Solid Edge part; units mm, degrees
sketch "Sketch1" plane through (0, 0, 0) normal (0, 0, 1) x (1, 0, 0)
  line L0 (-2.5, -5.2) -> (-8.5417, -5.2)
  line L1 (-5, -8.6603) -> (-8.75, -15.1554)
  line L2 (-5, 8.6603) -> (-8.75, 15.1554)
  arc A0 (-8.5417, 5.2) -> (-5, 8.6603) centre (0, 0) cw
  line L3 (-2.5, 5.2) -> (-8.5417, 5.2)
  line L4 (-2.5, 5.2) -> (-2.5, -5.2)
  arc A1 (-5, -8.6603) -> (-8.5417, -5.2) centre (0, 0) cw
  arc A2 (-8.75, -15.1554) -> (-8.75, 15.1554) centre (0, 0) cw
extrude "Protrusion1" add sketch "Sketch1" along normal blind 1.6
sketch "Sketch2" plane through (-10, 0, 1.6) normal (0, 0, 1) x (0.5, 0.866, 0)
  arc A0 (-11.4096, -6.9355) -> (11.7112, 6.4132) centre (5, -8.6603) cw
  line L0 (9.4741, 1.3887) -> (11.7112, 6.4132)
  arc A1 (-5.9397, -7.5104) -> (9.4741, 1.3887) centre (5, -8.6603) cw
  line L1 (-11.4096, -6.9355) -> (-5.9397, -7.5104)
extrude "ProtrusiónExtruida_2" add sketch "Sketch2" along normal blind 1
mirror "Mirror1" about plane through (0, 0, 0.8) normal (0, 0, 1) of "ProtrusiónExtruida_2"
sketch "Sketch3" plane through (-10, 0, 1.6) normal (0, 0, 1) x (0.5, 0.866, 0)
  circle A0 centre (6.6141, -3.456) radius 0.4
  circle A1 centre (4.8821, -4.456) radius 0.4
  circle A2 centre (3.15, -5.456) radius 0.4
  circle A3 centre (1.4179, -6.456) radius 0.4
  circle A4 centre (-0.3141, -7.456) radius 0.4
extrude "Cutout1" cut sketch "Sketch3" against normal through all
Model file for the job. Use its own axes, mm. A direction names the side the tool comes from. Coordinates: 2 decimals unless noted, no trailing zeros. Write each loop counter-clockwise with the first axis right and the second up, starting at its lowest first coordinate (ties: lowest second). Pieces come first, ordered by that corner, then holes. Notation, with made-up numbers: (85, 9) - (120, 9) arc R20 cw to (120, 32) - close; hole circle Ø3 at (62, -13.5). An arc over 180 degrees is marked (long way). One line per question, with ' | ' between items. Start each with the question number.
Q1. Pull direction Y, two halves, no side cores. Call faces 1 (the face through (-9, 0, 0)), 2 (the face through (-6.849, -11.862, 0.789)), 3 (the face through (-2.5, 0, 1)), 4 (the face through (-7.01, 7.13, 0.79)): pulls with the +Y half, pulls with the -Y half, needs draft (parallel to the pull), parting line crosses it, or undercut.
Q2. Cut at C-C, the plane x = -7. List the corners of the cut face in (y, z), then the cut area to 3 significant figures.
Q3. Cut at A-A, the plane z = 1.1. List the corners of the cut face in (x, y).
Q4. Cut at B-B, the plane y = -2. List the corners of the cut face in (x, z).
Q5. 3-axis set-ups, long thin cutter, end or side, ignore diameter. For faces 5 (the face through (-11, 0, 2)), 6 (the face through (-16.5, -0.2, 2.1)), 7 (the face through (-8.105, 11.155, -0.493)), 8 (the face through (-11, 0.1, -0.5)): which of +Z, -Z, +X, -X, +Y, -Y reach the whole face in a straight line?
Q6. Pin check, flat tips, straight feed: pin 1 (2 mm diameter, centred on x = -11.5, z = 0, fed in from -Y); pin 2 (1.3 mm diameter, centred on x = -5, z = 1, fed in from +Y); pin 3 (1.5 mm diameter, centred on x = -5, z = -0.5, fed in from -Y). Stop position of each tip, or through.
Q7. Drill centre lines: line 1 (Y direction, x = -5.25, z = 0.8); line 2 (Z direction, x = -6.5, y = 2); line 3 (Y direction, x = -8.5, z = -0.6). Where is each one in solid material? Low to high. Write a range as [from, to].
Q8. Cut at D-D, the plane x = -15. List the corners of the cut face in (y, z).
Answer below:
1) face 1: undercut | face 2: pulls with the -Y half | face 3: needs draft | face 4: undercut
2) outline: (-12.12, 0) - (-9.63, 0) - (-9.63, -1) - (-8.49, -1) - (-8.49, 0) - (-7.14, 0) - (-7.14, 1.6) - (-8.49, 1.6) - (-8.49, 2.6) - (-9.63, 2.6) - (-9.63, 1.6) - (-12.12, 1.6) - close; (-5.2, 0) - (5.2, 0) - (5.2, 1.6) - (-5.2, 1.6) - close; (7.14, 0) - (8.49, 0) - (8.49, -1) - (9.63, -1) - (9.63, 0) - (12.12, 0) - (12.12, 1.6) - (9.63, 1.6) - (9.63, 2.6) - (8.49, 2.6) - (8.49, 1.6) - (7.14, 1.6) - close | area: 37.2 mm^2
3) outline: (-8.75, -15.16) - (-5, -8.66) arc R10 cw to (-8.54, -5.2) - (-2.5, -5.2) - (-2.5, 5.2) - (-8.54, 5.2) arc R10 cw to (-5, 8.66) - (-8.75, 15.16) arc R17.5 ccw to start; hole circle Ø0.8 at (-3.7, -4); hole circle Ø0.8 at (-3.7, -2); hole circle Ø0.8 at (-3.7, 0); hole circle Ø0.8 at (-3.7, 2); hole circle Ø0.8 at (-3.7, 4)
4) outline: (-17.39, 0) - (-16.38, 0) - (-16.38, -1) - (-10.82, -1) - (-10.82, 0) - (-4.1, 0) - (-4.1, 1.6) - (-10.82, 1.6) - (-10.82, 2.6) - (-16.38, 2.6) - (-16.38, 1.6) - (-17.39, 1.6) - close; (-3.3, 0) - (-2.5, 0) - (-2.5, 1.6) - (-3.3, 1.6) - close
5) face 5: +Z, +X | face 6: +Z, -X | face 7: -Z, +X, +Y | face 8: -Z, +X
6) pin 1: y = -14 | pin 2: y = 9.79 | pin 3: y = -9.63
7) line 1: [-9.09, -8.51], [-5.2, 5.2], [8.51, 9.09] | line 2: [0, 1.6] | line 3: [-11.7, -6.98], [6.98, 11.7]
8) outline: (-9.01, 0) - (-6.87, 0) - (-6.87, -1) - (6.87, -1) - (6.87, 0) - (9.01, 0) - (9.01, 1.6) - (6.87, 1.6) - (6.87, 2.6) - (-6.87, 2.6) - (-6.87, 1.6) - (-9.01, 1.6) - close
